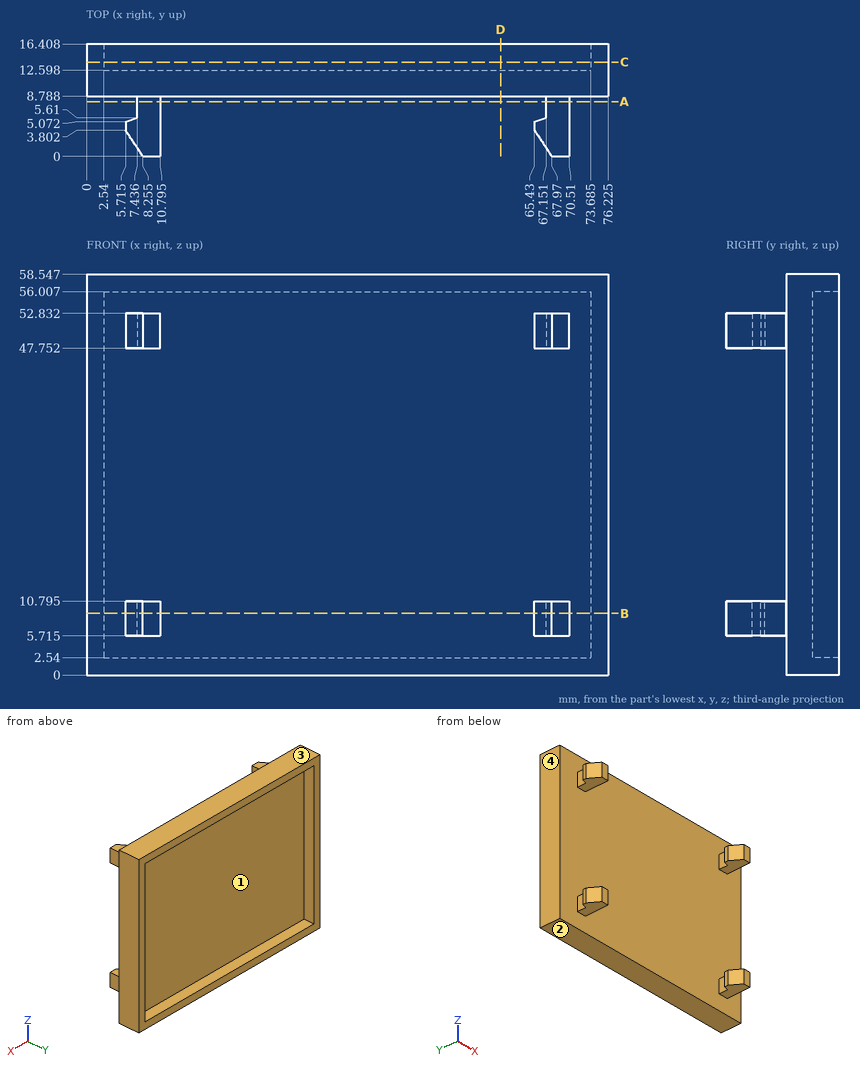
Source: three-view drawing plus pictorial views. Frame: mm from the lowest corner of the part. Give positions to 0.01 mm unless a question says otherwise; leave off trailing zeros. Order: outer loops, then holes, each group sorted by start corner. A loop starts at its lowest first (then second) coordinate and runs counter-clockwise, first axis right, second up. Notation, with made-up numbers: M 3.25,-3.5 L 45.25,-3.5 A36 ccw 45.25,35.5 Z; hole C 44.5,0 d8. An arc over 180 degrees is marked long. Return JSON: item names as keys, results as strings.
1) Section query C-C on y = 13.75. Output: boundary loops of the cut face in (x, z) (1 decimal).
Taken from the geometry:
{"outline": "M 0,0 L 76.2,0 L 76.2,58.5 L 0,58.5 Z; hole M 2.5,2.5 L 73.7,2.5 L 73.7,56 L 2.5,56 Z"}
2) Section query B-B on z = 9. Output: boundary loops of the cut face in (x, y) (1 decimal).
Taken from the geometry:
{"outline": "M 0,8.8 L 7.4,8.8 L 7.4,5.6 L 5.7,5.1 L 5.7,3.8 L 8.3,0 L 10.8,0 L 10.8,8.8 L 67.2,8.8 L 67.2,5.6 L 65.4,5.1 L 65.4,3.8 L 68,0 L 70.5,0 L 70.5,8.8 L 76.2,8.8 L 76.2,16.4 L 73.7,16.4 L 73.7,12.6 L 2.5,12.6 L 2.5,16.4 L 0,16.4 Z"}
3) Section query A-A on y = 8. Output: boundary loops of the cut face in (x, z) (1 decimal).
Taken from the geometry:
{"outline": "M 7.4,5.7 L 10.8,5.7 L 10.8,10.8 L 7.4,10.8 Z; M 7.4,47.8 L 10.8,47.8 L 10.8,52.8 L 7.4,52.8 Z; M 67.2,5.7 L 70.5,5.7 L 70.5,10.8 L 67.2,10.8 Z; M 67.2,47.8 L 70.5,47.8 L 70.5,52.8 L 67.2,52.8 Z"}
4) Section query D-D on x = 60.5. Output: boundary loops of the cut face in (y, z).
Taken from the geometry:
{"outline": "M 8.79,0 L 16.41,0 L 16.41,2.54 L 12.6,2.54 L 12.6,56.01 L 16.41,56.01 L 16.41,58.55 L 8.79,58.55 Z"}
5) Line query: L1, parallel to X at y = 13.75, z = 12 (1 decimal); L2, parallel to Z at x = 40, y = 15.25; L3, parallel to X at y = 4.5, z = 49.5 (1 decimal). Output: solid intervals per line, ascending. Write a range as [from, to].
Taken from the geometry:
{"L1": "x = [0, 2.5], [73.7, 76.2]", "L2": "z = [0, 2.54], [56.01, 58.55]", "L3": "x = [5.7, 10.8], [65.4, 70.5]"}
6) Mould query, pull axis Z, two halves, no side actions, for the marked faces 1, 2, 3 and 4. Classes: released by +Z, released by -Z, zero draft, split by the parting line, or undercut.
Taken from the geometry:
{"face 1": "undercut", "face 2": "released by -Z", "face 3": "released by +Z", "face 4": "zero draft"}
7) Contact query for flat-ended pins moving along their axis: pin 1 (1.6 mm diameter, centred on y = 7, z = 8, fed in from -X); pin 2 (2.5 mm diameter, centred on x = 9.5, y = 3, fed in from +Z); pin 3 (1.5 mm diameter, centred on x = 7.5, y = 3, fed in from -Z) (3 decimals); pin 4 (4 mm diameter, centred on y = 6, z = 45.5, fed in from +X). Output: stop coordinate, or through.
Taken from the geometry:
{"pin 1": "stops at x = 7.44", "pin 2": "stops at z = 52.83", "pin 3": "stops at z = 5.715", "pin 4": "passes through"}
